```python
from build123d import *

# Parameters (mm, degrees)
ESBO_O1_R                = 12.7
RESSALTO_EXTRUS_O1_DEPTH = 45
FILETE1_R                = 1
ESBO_O2_R                = 1
RESSALTO_EXTRUS_O2_DEPTH = 4


with BuildPart() as part:
    # Esboço1 → Ressalto-extrusão1 (new body)
    with BuildSketch(Plane(origin=(0, 0, 0), x_dir=(1, 0, 0), z_dir=(0, 1, 0))):
        with Locations(Location((0, 0, 0), (0, 0, 90))):
            Circle(ESBO_O1_R)
    extrude(amount=RESSALTO_EXTRUS_O1_DEPTH)

    # Filete1
    filete1_edges = [part.edges().sort_by_distance(p)[0] for p in [
        (0, 0, 12.7),
        (0, 45, 12.7),
    ]]
    fillet(filete1_edges, radius=FILETE1_R)

    # Esboço2 → Ressalto-extrusão2 (add)
    with BuildSketch(Plane(origin=(0, 45, 0), x_dir=(1, 0, 0), z_dir=(0, 1, 0))):
        with Locations(Location((5, 0, 0), (0, 0, 270))):
            Circle(ESBO_O2_R)
        with Locations(Location((-5, 0, 0), (0, 0, 270))):
            Circle(ESBO_O2_R)
    extrude(amount=RESSALTO_EXTRUS_O2_DEPTH)


solid = part.part
```
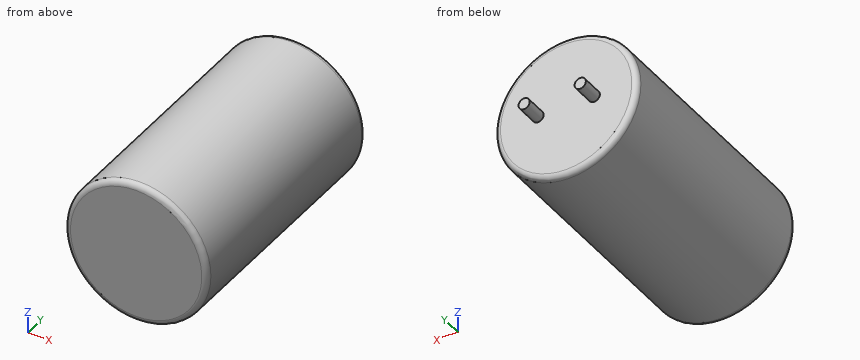
CAD build for the part. Positions are in the model's coordinates, mm. Coordinates: 2 decimals unless noted, no trailing zeros. Order: outer loops, then holes, each group sorted by start corner. A loop starts at its lowest first (then second) coordinate and runs counter-clockwise, first axis right, second up. Notation, with made-up numbers: (32.5, 33) - (54.5, 33) arc R25 ccw to (54.5, 64) - close; hole circle Ø10 at (28, -5). An arc over 180 degrees is marked (long way). Answer in a Markdown table with one row per item.
1. Slice it at B-B, the plane z = 0. List the corners of the cut face in (x, y).
Answer:
| item | result |
|---|---|
| outline | (-12.7, 1) arc R1 ccw to (-11.7, 0) - (11.7, 0) arc R1 ccw to (12.7, 1) - (12.7, 44) arc R1 ccw to (11.7, 45) - (6, 45) - (6, 49) - (4, 49) - (4, 45) - (-4, 45) - (-4, 49) - (-6, 49) - (-6, 45) - (-11.7, 45) arc R1 ccw to (-12.7, 44) - close |
2. Flat gauge pins, fed straight in: P1, Ø8, axis at x = -5.5, y = 24, coming from the -Z side; P2, Ø5, axis at y = 23.5, z = -9, coming from the +X side; P3, Ø2, axis at x = -1.5, z = 2, coming from the +Y side. Where does each tip first touch, or does it go through?
Answer:
| item | result |
|---|---|
| P1 | z = -12.61 |
| P2 | x = 10.91 |
| P3 | y = 45 |
3. Drill centre lines: L1, parallel to Y at x = 1, z = -0.25; L2, parallel to Z at x = 0.5, y = 14; L3, parallel to X at y = 16.5, z = -4. Where is each one in solid material? Low to high. Write a range as from..to.
Answer:
| item | result |
|---|---|
| L1 | 0..45 |
| L2 | -12.69..12.69 |
| L3 | -12.05..12.05 |
4. Slice it at C-C, the plane y = 35.5. List the corners of the cut face in (x, z).
Answer:
| item | result |
|---|---|
| outline | circle Ø25.4 at (0, 0) |
5. Slice it at A-A, the plane y = 46.5. List the corners of the cut face in (x, z), then the cut area to 3 significant figures.
Answer:
| item | result |
|---|---|
| outline | circle Ø2 at (-5, 0); circle Ø2 at (5, 0) |
| area | 6.28 mm² |
